Source: three-view drawing plus pictorial views. Frame: mm from the lowest corner of the part. Round coordinates to 2 decimals unless told otherwise and drop trailing zeros. Order: outer loops, then holes, each group sorted by start corner. A loop starts at its lowest first (then second) coordinate and runs counter-clockwise, first axis right, second up. Notation, with made-up numbers: (80.25, -10.75) - (112.25, -10.75) arc R25 cw to (112.25, 15.25) - close; hole circle Ø10 at (51, 81). An arc over 180 degrees is marked (long way). One line per item, written item: value. Start each with the question number.
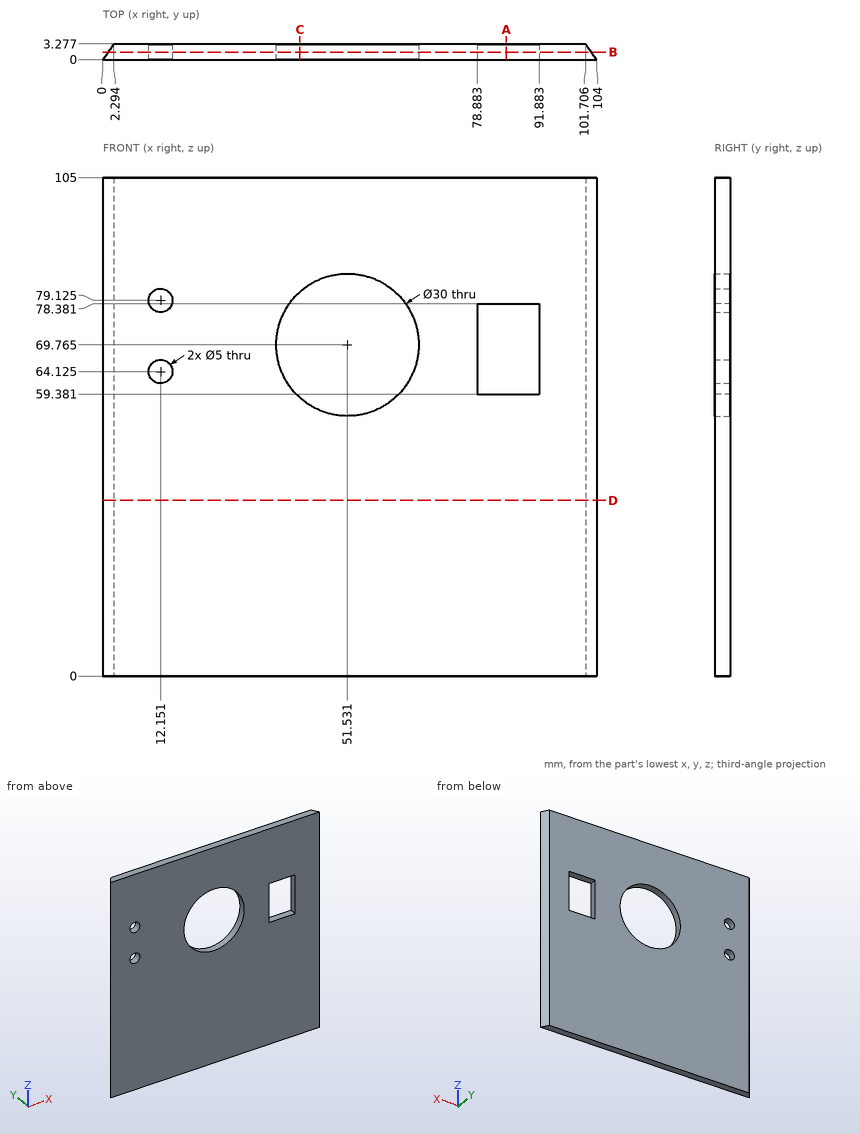
Item 1: First-contact query: pin 1 Ø1 at (y, z) = (1, 20.5) entering from -X; pin 2 Ø4 at (x, z) = (12.15, 64.12) entering from +Y. Flat tips, straight axial feed; report the tip coordinate or a pass-through.
Item 2: Section query B-B on y = 1.55. Return loops of the section in (x, z) (1 decimal).
Item 3: Section query C-C on x = 41.5. Return loops of the section in (y, z), and give its area (3 significant figures).
Item 4: Section query A-A on x = 85. Return loops of the section in (y, z).
Item 5: Line query: L1, parallel to Z at x = 12, y = 2.45; L2, parallel to X at y = 0.8, z = 77 (1 decimal); L3, parallel to Z at x = 79, y = 2.1. Output: solid intervals per line, ascending.
Item 6: Section query D-D on z = 37. Return loops of the section in (x, y) (1 decimal).
Geometry results:
1. pin 1: stops at x = 0.35
1. pin 2: passes through
2. outline: (1.1, 0) - (102.9, 0) - (102.9, 105) - (1.1, 105) - close; hole circle Ø5 at (12.2, 64.1); hole circle Ø5 at (12.2, 79.1); hole circle Ø30 at (51.5, 69.8); hole (78.9, 59.4) - (91.9, 59.4) - (91.9, 78.4) - (78.9, 78.4) - close
3. outline: (0, 0) - (3.28, 0) - (3.28, 58.61) - (0, 58.61) - close; (0, 80.92) - (3.28, 80.92) - (3.28, 105) - (0, 105) - close
3. area: 271 mm^2
4. outline: (0, 0) - (3.28, 0) - (3.28, 59.38) - (0, 59.38) - close; (0, 78.38) - (3.28, 78.38) - (3.28, 105) - (0, 105) - close
5. L1: z = 0 to 61.63, 66.62 to 76.63, 81.62 to 105
5. L2: x = 0.6 to 10.8, 13.5 to 38.4, 64.7 to 78.9, 91.9 to 103.4
5. L3: z = 0 to 59.38, 78.38 to 105
6. outline: (0, 0) - (104, 0) - (101.7, 3.3) - (2.3, 3.3) - close
